Autodesk Inventor part; units mm, degrees
ref_plane "YZ Plane" through (0, 0, 0) normal (1, 0, 0) x (0, 1, 0)
ref_plane "XZ Plane" through (0, 0, 0) normal (0, 1, 0) x (-1, 0, 0)
ref_plane "XY Plane" through (0, 0, 0) normal (0, 0, 1) x (1, 0, 0)
sketch "Sketch1" plane through (0, 0, 0) normal (0, 1, 0) x (-1, 0, 0)
  line L0 (-1.05, 6.1643) -> (-2.5, 6.1643)
  line L1 (-2.5, 6.1643) -> (-2.5, 1.1643)
  line L2 (-2.5, 1.1643) -> (-3.5, 1.1643)
  line L3 (-3.5, 1.1643) -> (-3.5, -3.8357)
  line L4 (-3.5, -3.8357) -> (-1.05, -3.8357)
  line L5 (0, -5.8357) -> (0, 8.1643)
  line L6 (-1.05, 6.1643) -> (-1.05, -3.8357)
  point P0 (0, 0)
  dimension "d0" = 5
  dimension "d1" = 5
  dimension "d3" = 1.05
  dimension "d4" = 2.5
  dimension "d5" = 3.5
revolve "Revolution1" add sketch "Sketch1" angle 360 about axis through (0, 0, -10) along (0, 0, 1)
sketch "Sketch2" plane through (0, 0, -3.8357) normal (0, 0, -1) x (-1, 0, 0)
  circle A0 centre (0, 0) radius 3.5
  line L0 (1.3478, 3.1911) -> (3.4375, 0.4283)
  line L1 (3.4375, 0.4283) -> (2.0897, -2.7628)
  line L2 (2.0897, -2.7628) -> (-1.3478, -3.1911)
  line L3 (-1.3478, -3.1911) -> (-3.4375, -0.4283)
  line L4 (-3.4375, -0.4283) -> (-2.0897, 2.7628)
  line L5 (-2.0897, 2.7628) -> (1.3478, 3.1911)
  circle A1 centre (0, 0) radius 5.601
  dimension "d8" = 7
  dimension "d10" = 6
extrude "Extrusion1" cut sketch "Sketch2" against normal blind 10 contours A0 | A1
fillet "Fillet2" radius 0.5 7 edges at (-2.7636, -1.1672, -3.8357) (-2.3927, 1.8097, -3.8357) (0.3709, 2.977, -3.8357) (2.7636, 1.1672, -3.8357) (2.3927, -1.8097, -3.8357) (-0.3709, -2.977, -3.8357) (-2.5, 0, 6.1643)
properties part number "Suction_electrode_cap"
Design review of the part built by this model. Coordinates are the model's own, in mm. A direction names the side the tool comes from. Coordinates: 2 decimals unless noted, no trailing zeros. Write each loop counter-clockwise with the first axis right and the second up, starting at its lowest first coordinate (ties: lowest second). Pieces come first, ordered by that corner, then holes.
1) Machinability: for faces 1 (the flat face through (2.4, -1.8, -1.1)), 2 (the cylindrical face through (-0.54, 2.44, 3.38)), which of the approach directions +Z, -Z, +X, -X, +Y, -Y give a long, thin tool a straight path to every point of the face, cutting with its end or side? Answer none if there is none.
2) To check wall thickness, follow L1, parallel to Y at x = 0, z = 2.25; L2, parallel to Z at x = -1.75, y = -2; L3, parallel to Y at x = 1.5, z = 5.5. State the ranges of each line that lie inside material, in increasing order.
3) Mouldability with a two-part tool opening along X and no side actions: class faces 3 (the flat face through (-2.4, 1.8, -1.1)), 4 (the cylindrical face through (1, -0.32, 1.09)), 5 (the flat face through (0, 1.2, -3.836)) as +X half, -X half, draft (parallel to the pull), parting line (faces both ways), or undercut.
4) Insertion check: pin 1 (1 mm diameter, centred on x = 0, z = -1, fed in from -Y); pin 2 (3 mm diameter, centred on x = -0.5, z = 4, fed in from -Y); pin 3 (3 mm diameter, centred on y = -1, z = 3, fed in from -X). Each pin has a flat end and moves straight along its axis. Give the tip position at first contact, or say it passes through.
5) Add section A-A (z = 5.25). Write out the cut boundary in (x, y).
Check result:
1. face 1: +Z, -Z, +X, -Y
1. face 2: +Z
2. L1: y = -2.5 to -1.05, 1.05 to 2.5
2. L2: z = -3.84 to 1.16
2. L3: y = -2 to 2
3. face 3: -X half
3. face 4: undercut
3. face 5: draft
4. pin 1: stops at y = -3.09
4. pin 2: stops at y = -2.5
4. pin 3: stops at x = -2.5
5. outline: circle Ø5 at (0, 0); hole circle Ø2.1 at (0, 0)
